Job drawing, mm, ordinate dimensions from the low corner. One solid piece. Coordinates: 2 decimals unless noted, no trailing zeros. Loops run counter-clockwise (first coordinate to the right, second up) from the corner with the lowest first, then second, coordinate; pieces in that order, holes last. Notation, with made-up numbers: (-13.5, -38) - (26.5, -38) arc R15 cw to (26.5, -21) - close; hole circle Ø7 at (33.25, 69). An arc over 180 degrees is marked (long way). Use a Markdown table: item, result. Add a question column.
1) Band-saw the part on B-B (y = 48). Give the cut face in (x, z).
2) Drop flat-ended pins along their axis: P1, Ø0.9, axis at y = 45.5, z = 2, coming from the +X side; P2, Ø6.5, axis at x = 5.5, y = 5.5, coming from the -Z side; P3, Ø1.5, axis at x = 3.5, z = 0.5, coming from the -Y side. Give the stop position or say it passes through.
3) Band-saw the part on C-C (z = 1.55). Give the cut face in (x, y), plus the area to 3 significant figures.
4) Band-saw the part on A-A (x = 5.75). Give the cut face in (y, z) (1 decimal).
5) Probe probe 1 along Y at (x, z) = (5.25, 2.7) (1 decimal); probe 2 along Y at (x, z) = (3.25, 1.7); probe 3 along X at (y, z) = (47.5, 0.6). List the from-to ranges inside material, lowest first. Write a range as [from, to].
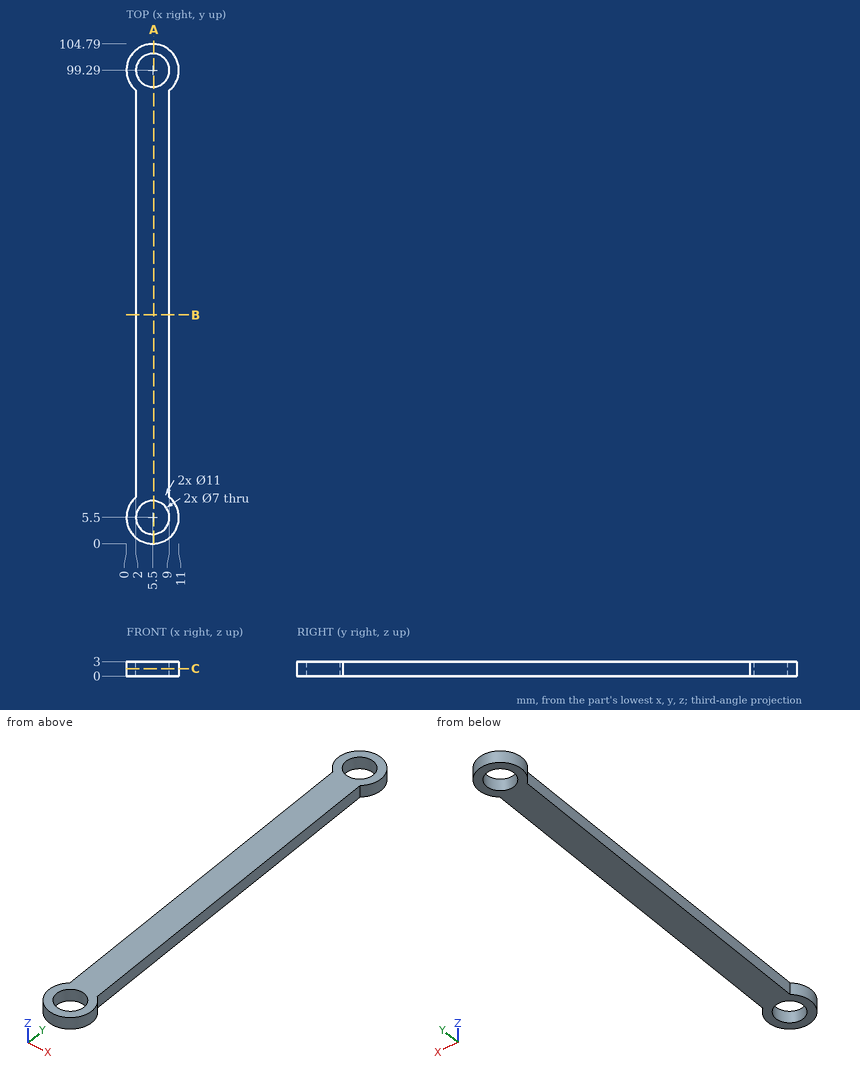
Answer block:
| question | item | result |
|---|---|---|
| 1 | outline | (2, 0) - (9, 0) - (9, 3) - (2, 3) - close |
| 2 | P1 | x = 9 |
| 2 | P2 | through |
| 2 | P3 | y = 0.14 |
| 3 | outline | (2, 9.74) arc R5.5 ccw (long way) to (9, 9.74) - (9, 95.05) arc R5.5 ccw (long way) to (2, 95.05) - close; hole circle Ø7 at (5.5, 5.5); hole circle Ø7 at (5.5, 99.29) |
| 3 | area | 698 mm2 |
| 4 | outline | (0, 0) - (2, 0) - (2, 3) - (0, 3) - close; (9, 0) - (95.8, 0) - (95.8, 3) - (9, 3) - close; (102.8, 0) - (104.8, 0) - (104.8, 3) - (102.8, 3) - close |
| 5 | probe 1 | [0, 2], [9, 95.8], [102.8, 104.8] |
| 5 | probe 2 | [0.48, 2.82], [8.18, 96.61], [101.97, 104.31] |
| 5 | probe 3 | [2, 9] |
